Geometry check sheet. Reference: the model listing, model coordinates, mm. Face numbers are marked on the shaded views. A direction names the side the tool comes from. Coordinates: 2 decimals unless noted, no trailing zeros. Write each loop counter-clockwise with the first axis right and the second up, starting at its lowest first coordinate (ties: lowest second). Pieces come first, ordered by that corner, then holes. Notation, with made-up numbers: (41, -27) -> (55, -27) arc R10 cw to (55, -15) -> close; hole circle Ø4 at (31, -37.75). An arc over 180 degrees is marked (long way). Put each result on its own line as item: value. Start each with the question number.
from build123d import *

# Parameters (mm, degrees)
EXTRUDE_2_DEPTH     = 6
SKETCH_2_R          = 4
EXTRUDE_3_DEPTH     = 6
EXTRUDE_4_DEPTH     = 6
SKETCH_5_R          = 27
CUT_EXTRUDE_2_DEPTH = 46.122056691
SKETCH_6_R          = 1.6
CUT_EXTRUDE_3_DEPTH = 46.122056691
FILLET_1_R          = 2
SKETCH_7_R          = 3.25
CUT_EXTRUDE_5_DEPTH = 3.5
FILLET_4_R          = 0.3
CUT_EXTRUDE_6_DEPTH = 6
CUT_EXTRUDE_7_DEPTH = 0.3


with BuildPart() as part:
    # 草图1 → 凸台-拉伸2 (new body)
    with BuildSketch(Plane.XY):
        with BuildLine():
            Line((-15, 25.980762114), (0, 0))
            Line((0, 0), (0, 30))
            ThreePointArc((0, 30), (-7.764571353, 28.977774789), (-15, 25.980762114))
        make_face()
    extrude(amount=EXTRUDE_2_DEPTH)

    # 草图2 → 凸台-拉伸3 (add)
    with BuildSketch(Plane.XY.offset(6)):
        with Locations((-3.656080302, 29.776384549)):
            Circle(SKETCH_2_R)
        with Locations((-11.721933855, 27.615145604)):
            Circle(SKETCH_2_R)
    extrude(amount=-EXTRUDE_3_DEPTH)

    # 草图4 → 凸台-拉伸4 (add, through all)
    with BuildSketch(Plane.XY.offset(6)):
        with BuildLine():
            Line((0, 0), (0, 40))
            ThreePointArc((0, 40), (-10.352761804, 38.637033052), (-20, 34.641016151))
            Line((-20, 34.641016151), (0, 0))
        make_face()
    extrude(amount=-EXTRUDE_4_DEPTH)

    # 草图5 → 切除-拉伸2 (cut, through all)
    with BuildSketch(Plane.XY.offset(6)):
        Circle(SKETCH_5_R)
    extrude(amount=-CUT_EXTRUDE_2_DEPTH, mode=Mode.SUBTRACT)

    # 草图6 → 切除-拉伸3 (cut, through all)
    with BuildSketch(Plane.XY.offset(6)):
        with Locations((-3.656080302, 29.776384549)):
            Circle(SKETCH_6_R)
        with Locations((-11.721933855, 27.615145604)):
            Circle(SKETCH_6_R)
    extrude(amount=-CUT_EXTRUDE_3_DEPTH, mode=Mode.SUBTRACT)

    # 圆角1
    fillet_1_edges = [part.edges().sort_by_distance(p)[0] for p in [
        (0, 40, 3),
        (-20, 34.641016151, 3),
    ]]
    fillet(fillet_1_edges, radius=FILLET_1_R)

    # 草图7 → 切除-拉伸5 (cut)
    with BuildSketch(Plane.XY.offset(6)):
        with Locations((-11.721933855, 27.615145604)):
            Circle(SKETCH_7_R)
        with Locations((-3.656080302, 29.776384549)):
            Circle(SKETCH_7_R)
    extrude(amount=-CUT_EXTRUDE_5_DEPTH, mode=Mode.SUBTRACT)

    # 圆角4
    fillet_4_edges = [part.edges().sort_by_distance(p)[0] for p in [
        (-2.110567489, 26.91738295, 4.25),
        (-4.464029693, 26.628414127, 4.25),
        (-9.448243946, 25.292897943, 4.25),
        (-11.630886413, 24.366421183, 4.25),
    ]]
    fillet(fillet_4_edges, radius=FILLET_4_R)

    # 草图8 → 切除-拉伸6 (cut)
    with BuildSketch(Plane.XY.offset(6)):
        with BuildLine():
            Line((-15.699530186, 27.192383937), (-14.076854363, 24.381826968))
            ThreePointArc((-14.076854363, 24.381826968), (-15.18603547, 25.615145604), (-15.699530186, 27.192383937))
        make_face()
        with BuildLine():
            Line((0, 31.399060372), (0, 28.153708727))
            ThreePointArc((0, 28.153708727), (0.343919698, 29.776384549), (0, 31.399060372))
        make_face()
    extrude(amount=-CUT_EXTRUDE_6_DEPTH, mode=Mode.SUBTRACT)

    # 草图9 → 切除-拉伸7 (cut)
    with BuildSketch(Plane.XY.offset(6)):
        with BuildLine():
            Line((0, 27), (0, 37.947331922))
            ThreePointArc((0, 37.947331922), (-0.623505597, 39.398284422), (-2.105263158, 39.944559918))
            ThreePointArc((-2.105263158, 39.944559918), (-10.352761804, 38.637033052), (-18.149068583, 35.645635211))
            ThreePointArc((-18.149068583, 35.645635211), (-19.159170525, 34.431667974), (-18.973665961, 32.86335345))
            Line((-18.973665961, 32.86335345), (-13.5, 23.382685902))
            ThreePointArc((-13.5, 23.382685902), (-13.010612738, 23.658485924), (-12.515593512, 23.924044788))
            ThreePointArc((-12.515593512, 23.924044788), (-12.356405623, 24.222223556), (-12.575834101, 24.479327629))
            ThreePointArc((-12.575834101, 24.479327629), (-12.991810022, 30.606786377), (-8.873046225, 26.051067832))
            ThreePointArc((-8.873046225, 26.051067832), (-8.840528862, 25.714624698), (-8.515455807, 25.622002506))
            ThreePointArc((-8.515455807, 25.622002506), (-6.988114218, 26.07999731), (-5.436400199, 26.447032969))
            ThreePointArc((-5.436400199, 26.447032969), (-5.201189771, 26.689782668), (-5.341250476, 26.997409651))
            ThreePointArc((-5.341250476, 26.997409651), (-4.052155668, 33.002159542), (-1.348672009, 27.487636645))
            ThreePointArc((-1.348672009, 27.487636645), (-1.410150609, 27.155263747), (-1.123200469, 26.976627304))
            ThreePointArc((-1.123200469, 26.976627304), (-0.561721812, 26.994156194), (0, 27))
        make_face()
    extrude(amount=-CUT_EXTRUDE_7_DEPTH, mode=Mode.SUBTRACT)


solid = part.part
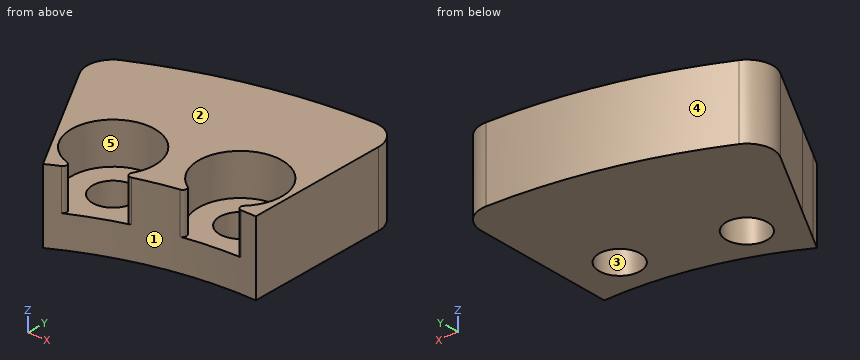
Item 1: Go/stop test with flat-tipped pins: P1, Ø1.5, axis at x = -4.5, z = 2, coming from the -Y side; P2, Ø2, axis at x = -10, z = 5, coming from the +Y side; P3, Ø1.9, axis at x = -3.66, y = 29.78, coming from the +Z side; P4, Ø5, axis at x = -3.66, y = 29.78, coming from the +Z side. Record where each tip stops, or that it passes through.
Item 2: Mould release check, pull along X, two halves, no side actions. Record for the marked faces 1, 2 and 3: released by +X, released by -X, zero draft, split by the parting line, or undercut.
Item 3: Scan lines: line 1 along X through (y, z) = (30.25, 3.7); line 2 along X through (y, z) = (28.5, 2.35); line 3 along Y through (x, z) = (-12.25, 0.7). Record each from-to range of solid material in increasing order. Write a range as [from, to].
Item 4: Section check C-C, the plane z = 2.2. Enter the section's corners in (x, y).
Item 5: Section check A-A, the plane x = -2.5. Enter the section's corners in (y, z).
Item 6: Section check B-B, the plane y = 28.75. Enter the section's corners in (x, z), and give its area (3 significant figures).
Item 7: Access from +Z, -Z, +X, -X, +Y, -Y to the whole of each face (thin tool, end or side, straight path). Record for the marked faces 4 and 5.
Item 8: Section check D-D, the plane y = 25.25. Enter the section's corners in (x, z), and give its area (3 significant figures).
From the geometry:
1. P1: y = 26.48
1. P2: y = 38.97
1. P3: through
1. P4: z = 2.5
2. face 1: released by +X
2. face 2: zero draft
2. face 3: undercut
3. line 1: [-17.46, -13.62], [-9.82, -6.87], [-0.44, 0]
3. line 2: [-16.45, -13.05], [-10.39, -4.62], [-2.69, 0]
3. line 3: [24.06, 26.1], [29.13, 38.08]
4. outline: (-18.97, 32.86) -> (-13.5, 23.38) arc R27 cw to (0, 27) -> (0, 37.95) arc R2 ccw to (-2.11, 39.94) arc R40 ccw to (-18.15, 35.65) arc R2 ccw to start; hole circle Ø3.2 at (-11.72, 27.62); hole circle Ø3.2 at (-3.66, 29.78)
5. outline: (26.88, 0) -> (28.67, 0) -> (28.67, 2.5) -> (26.88, 2.5) -> close; (30.88, 0) -> (39.92, 0) -> (39.92, 5.7) -> (32.81, 5.7) -> (32.81, 2.5) -> (30.88, 2.5) -> close
6. outline: (-16.6, 0) -> (-12.85, 0) -> (-12.85, 2.5) -> (-14.77, 2.5) -> (-14.77, 5.7) -> (-16.6, 5.7) -> close; (-10.59, 0) -> (-4.88, 0) -> (-4.88, 2.5) -> (-6.74, 2.5) -> (-6.74, 5.7) -> (-8.68, 5.7) -> (-8.68, 2.5) -> (-10.59, 2.5) -> close; (-2.43, 0) -> (0, 0) -> (0, 5.7) -> (-0.57, 5.7) -> (-0.57, 2.5) -> (-2.43, 2.5) -> close
6. area: 43.6 mm²
7. face 4: +Z, -Z, -X, +Y
7. face 5: +Z
8. outline: (-14.58, 0) -> (-9.56, 0) -> (-9.56, 2.5) -> (-13.95, 2.5) -> (-13.95, 5.7) -> (-14.58, 5.7) -> close
8. area: 14.5 mm²
